```python
from build123d import *

# Parameters (mm, degrees)
SKETCH_1_W     = 38
SKETCH_1_H     = 4
CHAMFER_1_SIZE = 1


with BuildPart() as part:
    # 草图1 → 旋转1 (revolve)
    with BuildSketch(Plane.XY, mode=Mode.PRIVATE) as revolve_1_sk:
        Polygon((0, 0), (0, 4), (15, 4), (15, 5), (45, 5), (45, 6), (345, 6), (345, 5), (352.9, 5), (352.9, 4.8), (353.7, 4.8), (353.7, 5), (357, 5), (357, 0), align=None)
        with Locations((376, 2)):
            Rectangle(SKETCH_1_W, SKETCH_1_H)
    revolve(revolve_1_sk.sketch.rotate(Axis((0, 0, 0), (1, 0, 0)), 90), axis=Axis((0, 0, 0), (1, 0, 0)))

    # 倒角1
    chamfer_1_edges = [part.edges().sort_by_distance(p)[0] for p in [
        (0, 0, -4),
        (15, 0, -5),
        (357, 0, -5),
        (395, 0, -4),
    ]]
    chamfer(chamfer_1_edges, length=CHAMFER_1_SIZE - 0.0001)  # a hair under: the kernel refuses the full size


solid = part.part
```
Could you check a few things on this model? Use its own coordinates, in mm. A direction names the side the tool comes from. Round coordinates to 2 decimals unless told otherwise and drop trailing zeros. Loops run counter-clockwise (first coordinate to the right, second up) from the corner with the lowest first, then second, coordinate; pieces in that order, holes last. Notation, with made-up numbers: (7.5, 20) - (49.5, 20) arc R10 cw to (49.5, 36) - close; hole circle Ø9 at (53.25, 55.25). An arc over 180 degrees is marked (long way). Answer in a Markdown table with one row per item. Add a question column.
(1) I need wall thicknesses on line 1 along Z through (x, y) = (232, -0.25); line 2 along Z through (x, y) = (205, -3.5); line 3 along X through (y, z) = (-3.25, 4.75). Which ranges of each line are inside material? Lowest first, please.
(2) I'm going to push flat-ended pins straight in: pin 1 (5 mm diameter, centred on x = 82, z = 4.5, fed in from -Y); pin 2 (4 mm diameter, centred on x = 127.5, y = -4.5, fed in from +Z); pin 3 (3 mm diameter, centred on x = 145, z = 4.5, fed in from -Y). Where does each tip first touch, or does it pass through?
(3) If we section it at B-B (x = 84): Please give me the cut outline in (y, z), plus the area to 3 significant figures.
(4) For faces 1 (the face through (31, 0, -5)), 2 (the face through (197.1, -1.802, 5.723)), which set-ups out of +Z, -Z, +X, -X, +Y, -Y let a thin tool reach every point of the face, with its end or its side?
(5) If we section it at A-A (x = 369): Please give me the cut outline in (y, z).
Model answer:
| question | item | result |
|---|---|---|
| 1 | line 1 | z = -5.99 to 5.99 |
| 1 | line 2 | z = -4.87 to 4.87 |
| 1 | line 3 | x = 45 to 345 |
| 2 | pin 1 | stops at y = -5.66 |
| 2 | pin 2 | stops at z = 5.45 |
| 2 | pin 3 | stops at y = -5.2 |
| 3 | outline | circle Ø12 at (0, 0) |
| 3 | area | 113 mm² |
| 4 | face 1 | -X |
| 4 | face 2 | +X, -X |
| 5 | outline | circle Ø8 at (0, 0) |
